Geometry check sheet. Reference: the model listing, model coordinates, mm. Face numbers are marked on the shaded views. A direction names the side the tool comes from. Coordinates: 2 decimals unless noted, no trailing zeros. Order: outer loops, then holes, each group sorted by start corner. A loop starts at its lowest first (then second) coordinate and runs counter-clockwise, first axis right, second up.
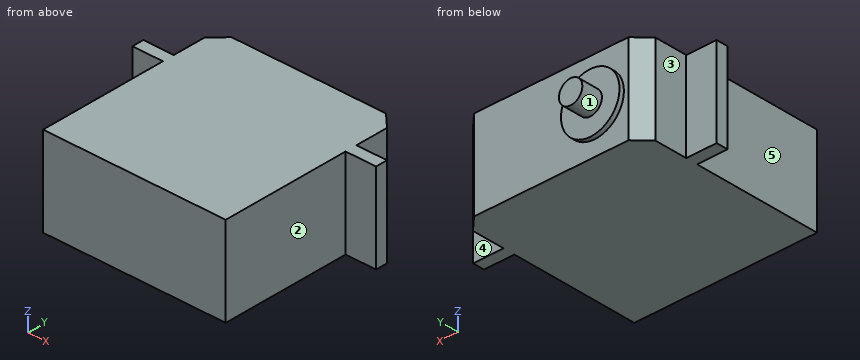
```python
from build123d import *

# Parameters (mm, degrees)
SKETCH1_W           = 39
SKETCH1_H           = 19
BOSS_EXTRUDE1_DEPTH = 40
SKETCH2_W           = 19
SKETCH2_H           = 2.5
BOSS_EXTRUDE2_DEPTH = 6.5
SKETCH3_W           = 19
SKETCH3_H           = 2.5
BOSS_EXTRUDE3_DEPTH = 6.5
SKETCH4_R           = 6.25
BOSS_EXTRUDE4_DEPTH = 1
SKETCH5_R           = 2.5
BOSS_EXTRUDE5_DEPTH = 4.5
CHAMFER1_SIZE       = 3
CHAMFER2_SIZE       = 3


with BuildPart() as part:
    # Sketch1 → Boss-Extrude1 (new body)
    with BuildSketch(Plane(origin=(0, 0, 0), x_dir=(1, 0, 0), z_dir=(0, 1, 0))):
        with Locations((19.5, 9.5)):
            Rectangle(SKETCH1_W, SKETCH1_H)
    extrude(amount=BOSS_EXTRUDE1_DEPTH)

    # Sketch2 → Boss-Extrude2 (add)
    with BuildSketch(Plane(origin=(39, 0, 0), x_dir=(0, 0, -1), z_dir=(1, 0, 0))):
        with Locations((9.5, 28.75)):
            Rectangle(SKETCH2_W, SKETCH2_H)
    extrude(amount=BOSS_EXTRUDE2_DEPTH)

    # Sketch3 → Boss-Extrude3 (add)
    with BuildSketch(Plane.ZY):
        with Locations((-9.5, 28.75)):
            Rectangle(SKETCH3_W, SKETCH3_H)
    extrude(amount=BOSS_EXTRUDE3_DEPTH)

    # Sketch4 → Boss-Extrude4 (add)
    with BuildSketch(Plane(origin=(0, 40, 0), x_dir=(1, 0, 0), z_dir=(0, 1, 0))):
        with Locations(Location((10.25, 9.5, 0), (0, 0, 90))):
            Circle(SKETCH4_R)
    extrude(amount=BOSS_EXTRUDE4_DEPTH)

    # Sketch5 → Boss-Extrude5 (add)
    with BuildSketch(Plane(origin=(0, 41, 0), x_dir=(1, 0, 0), z_dir=(0, 1, 0))):
        with Locations(Location((10.25, 9.5, 0), (0, 0, 270))):
            Circle(SKETCH5_R)
    extrude(amount=BOSS_EXTRUDE5_DEPTH)

    # Chamfer1
    chamfer1_edges = [part.edges().sort_by_distance(p)[0] for p in [
        (0, 40, -9.5),
    ]]
    chamfer(chamfer1_edges, length=CHAMFER1_SIZE)

    # Chamfer2
    chamfer2_edges = [part.edges().sort_by_distance(p)[0] for p in [
        (39, 40, -9.5),
    ]]
    chamfer(chamfer2_edges, length=CHAMFER2_SIZE)


solid = part.part
```
Item 1: Sectioned sample at A-A (z = -2.25). Record the cut outline in (x, y).
Item 2: Sectioned sample at C-C (z = -9.5). Record the cut outline in (x, y).
Item 3: Sectioned sample at D-D (y = 7). Record the cut outline in (x, z).
Item 4: Tool access check on the marked faces 1, 2, 3, 4 and 5. Record the directions out of +Z, -Z, +X, -X, +Y, -Y that give a thin tool (end or side, any length) a straight path to the whole face; none if there is none.
Item 5: Depth check by flat-ended pin: P1, Ø2, axis at x = -4.5, z = -6.5, coming from the +Y side; P2, Ø3, axis at x = -2.5, z = -9, coming from the -Y side; P3, Ø7.5, axis at y = 34.5, z = -9.5, coming from the -X side. Enter the tip coordinate at first touch or a pass-through.
Item 6: Sectioned sample at B-B (x = 10.25). Record the cut outline in (y, z), and give its area (3 significant figures).
Item 7: Thickness scan on line 1 along X through (y, z) = (36, -1); line 2 along Y through (x, z) = (21, -2); line 3 along Y through (x, z) = (14, -4.75). Record the ranges inside material, lowest first.
Geometry check:
1. outline: (-6.5, 27.5) - (0, 27.5) - (0, 0) - (39, 0) - (39, 27.5) - (45.5, 27.5) - (45.5, 30) - (39, 30) - (39, 37) - (36, 40) - (3, 40) - (0, 37) - (0, 30) - (-6.5, 30) - close
2. outline: (-6.5, 27.5) - (0, 27.5) - (0, 0) - (39, 0) - (39, 27.5) - (45.5, 27.5) - (45.5, 30) - (39, 30) - (39, 37) - (36, 40) - (16.5, 40) - (16.5, 41) - (12.75, 41) - (12.75, 45.5) - (7.75, 45.5) - (7.75, 41) - (4, 41) - (4, 40) - (3, 40) - (0, 37) - (0, 30) - (-6.5, 30) - close
3. outline: (0, -19) - (39, -19) - (39, 0) - (0, 0) - close
4. face 1: +Y
4. face 2: +Z, -Z, +X, -Y
4. face 3: +Z, -Z, -X, +Y
4. face 4: +Z, -Z, +X, +Y
4. face 5: +Z, -Z, -X, -Y
5. P1: stops at y = 30
5. P2: stops at y = 27.5
5. P3: stops at x = 0
6. outline: (0, -19) - (40, -19) - (40, -15.75) - (41, -15.75) - (41, -12) - (45.5, -12) - (45.5, -7) - (41, -7) - (41, -3.25) - (40, -3.25) - (40, 0) - (0, 0) - close
6. area: 795 mm2
7. line 1: x = 0 to 39
7. line 2: y = 0 to 40
7. line 3: y = 0 to 41
